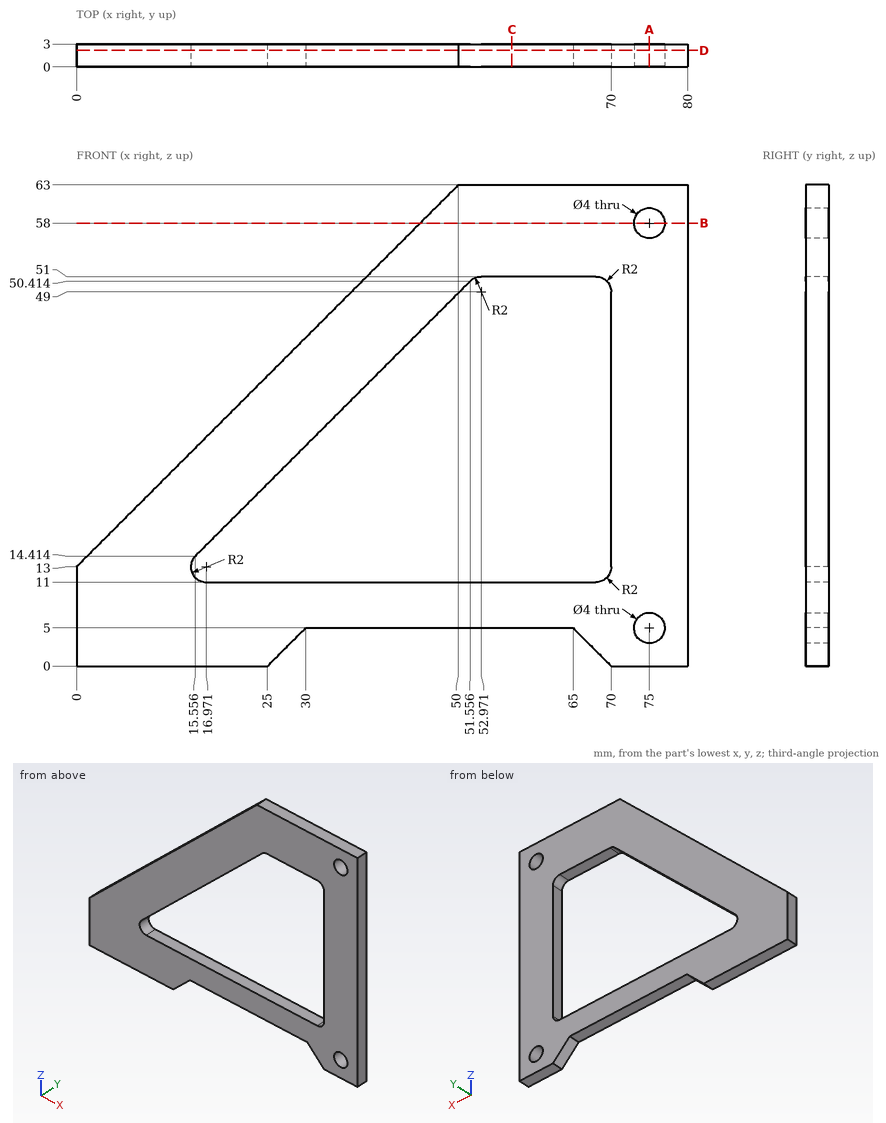
Design review of the part shown in the three views and the two pictorial views. Dimensions are in mm from the part's minimum x, y and z. Round coordinates to 2 decimals unless told otherwise and drop trailing zeros. Write each loop counter-clockwise with the first axis right and the second up, starting at its lowest first coordinate (ties: lowest second). Pieces come first, ordered by that corner, then holes. Notation, with made-up numbers: (-6.5, 55) - (49.5, 55) arc R32 cw to (49.5, 87) - close; hole circle Ø10 at (45, 71). An arc over 180 degrees is marked (long way). Return JSON: item names as keys, results as strings. Group by question number.
Item 1: We need section A-A on x = 75. Write out the cut boundary in (y, z), and give its area (3 significant figures).
Item 2: We need section C-C on x = 57. Write out the cut boundary in (y, z), and give its area (3 significant figures).
Item 3: Insertion check: P1, Ø0.9, axis at x = 46.5, y = 2, coming from the -Z side; P2, Ø1, axis at y = 2.5, z = 50.5, coming from the -X side; P3, Ø6.5, axis at x = 75, z = 58, coming from the -Y side; P4, Ø1.5, axis at y = 2, z = 38, coming from the -X side. Each pin has a flat end and moves straight along its axis. Give the tip position at first contact, or say it passes through.
Item 4: We need section B-B on z = 58. Write out the cut boundary in (x, y).
Item 5: We need section D-D on y = 2.15. Write out the cut boundary in (x, z) (1 decimal), and give its area (3 significant figures).
Item 6: For probe 1 along Z at (x, y) = (75, 1.2); probe 2 along Z at (x, y) = (55, 2.3); probe 3 along X at (y, z) = (0.8, 34), list the stretches that pass through material, from the lowest coordinate up. Write a range as [from, to].
Model answer:
{
 "1": {"outline": "(0, 0) - (3, 0) - (3, 3) - (0, 3) - close; (0, 7) - (3, 7) - (3, 56) - (0, 56) - close; (0, 60) - (3, 60) - (3, 63) - (0, 63) - close", "area": "165 mm²"},
 "2": {"outline": "(0, 5) - (3, 5) - (3, 11) - (0, 11) - close; (0, 51) - (3, 51) - (3, 63) - (0, 63) - close", "area": "54.0 mm²"},
 "3": {"P1": "stops at z = 5", "P2": "stops at x = 37", "P3": "stops at y = 0", "P4": "stops at x = 24.25"},
 "4": {"outline": "(45, 0) - (73, 0) - (73, 3) - (45, 3) - close; (77, 0) - (80, 0) - (80, 3) - (77, 3) - close"},
 "5": {"outline": "(0, 0) - (25, 0) - (30, 5) - (65, 5) - (70, 0) - (80, 0) - (80, 63) - (50, 63) - (0, 13) - close; hole (15.6, 14.4) arc R2 ccw to (17, 11) - (68, 11) arc R2 ccw to (70, 13) - (70, 49) arc R2 ccw to (68, 51) - (53, 51) arc R2 ccw to (51.6, 50.4) - close; hole circle Ø4 at (75, 5); hole circle Ø4 at (75, 58)", "area": "2,060 mm²"},
 "6": {"probe 1": "z = [0, 3], [7, 56], [60, 63]", "probe 2": "z = [5, 11], [51, 63]", "probe 3": "x = [21, 35.14], [70, 80]"}
}
